```python
from build123d import *

# Parameters (mm, degrees)
BOSS_EXTRUDE1_DEPTH = 20
FILLET1_R           = 5
SKETCH2_R           = 30
BOSS_EXTRUDE2_DEPTH = 5
SKETCH3_R           = 17.5
BOSS_EXTRUDE3_DEPTH = 10
SKETCH4_R           = 21.75
BOSS_EXTRUDE4_DEPTH = 10
CHAMFER1_SIZE       = 5


with BuildPart() as part:
    # Sketch1 → Boss-Extrude1 (new body)
    with BuildSketch(Plane.XY):
        with BuildLine():
            Line((-32.88854382, 29.22291236), (-27.763932023, 39.472135955))
            ThreePointArc((-27.763932023, 39.472135955), (-24.076971234, 43.506508084), (-18.819660113, 45))
            Line((-18.819660113, 45), (18.819660113, 45))
            ThreePointArc((18.819660113, 45), (24.076971234, 43.506508084), (27.763932023, 39.472135955))
            Line((27.763932023, 39.472135955), (32.88854382, 29.22291236))
            ThreePointArc((32.88854382, 29.22291236), (34.464979789, 24.873698861), (35, 20.27864045))
            Line((35, 20.27864045), (35, -20.27864045))
            ThreePointArc((35, -20.27864045), (34.464979789, -24.873698861), (32.88854382, -29.22291236))
            Line((32.88854382, -29.22291236), (27.763932023, -39.472135955))
            ThreePointArc((27.763932023, -39.472135955), (24.076971234, -43.506508084), (18.819660113, -45))
            Line((18.819660113, -45), (-18.819660113, -45))
            ThreePointArc((-18.819660113, -45), (-24.076971234, -43.506508084), (-27.763932023, -39.472135955))
            Line((-27.763932023, -39.472135955), (-32.88854382, -29.22291236))
            ThreePointArc((-32.88854382, -29.22291236), (-34.464979789, -24.873698861), (-35, -20.27864045))
            Line((-35, -20.27864045), (-35, 20.27864045))
            ThreePointArc((-35, 20.27864045), (-34.464979789, 24.873698861), (-32.88854382, 29.22291236))
        make_face()
    extrude(amount=BOSS_EXTRUDE1_DEPTH)

    # Fillet1
    fillet1_edges = [part.edges().sort_by_distance(p)[0] for p in [
        (24.076971234, -43.506508084, 20),
        (30.326237921, -34.347524158, 20),
        (34.464979789, -24.873698861, 20),
        (35, 0, 20),
        (34.464979789, 24.873698861, 20),
        (30.326237921, 34.347524158, 20),
        (24.076971234, 43.506508084, 20),
        (0, 45, 20),
        (-24.076971234, 43.506508084, 20),
        (-30.326237921, 34.347524158, 20),
        (-24.076971234, -43.506508084, 20),
        (-34.464979789, 24.873698861, 20),
        (-35, 0, 20),
        (-34.464979789, -24.873698861, 20),
        (-30.326237921, -34.347524158, 20),
        (0, -45, 20),
    ]]
    fillet(fillet1_edges, radius=FILLET1_R)

    # Sketch2 → Boss-Extrude2 (add)
    with BuildSketch(Plane.XY.offset(20)):
        Circle(SKETCH2_R)
    extrude(amount=BOSS_EXTRUDE2_DEPTH)

    # Sketch3 → Boss-Extrude3 (add)
    with BuildSketch(Plane.XY.offset(25)):
        Circle(SKETCH3_R)
    extrude(amount=BOSS_EXTRUDE3_DEPTH)

    # Sketch4 → Boss-Extrude4 (add)
    with BuildSketch(Plane.XY.offset(35)):
        Circle(SKETCH4_R)
    extrude(amount=BOSS_EXTRUDE4_DEPTH)

    # Chamfer1
    # the kernel refuses this chamfer: 5 mm, written as the material it adds along each edge
    with BuildSketch(Plane(origin=(0, 0, 35), x_dir=(1, 0, 0), z_dir=(0, -1, 0))) as chamfer1_piece_1_section:
        Polygon((17.5 + CHAMFER1_SIZE, 0), (17.5, -CHAMFER1_SIZE), (17.5, 0), align=None)
    chamfer1_piece_1 = revolve(axis=Axis((0, 0, 35), (0, 0, 1)), mode=Mode.PRIVATE)
    chamfer1_piece_1 = chamfer1_piece_1 & Plane(origin=(0, 0, 32.136850645), x_dir=(1, 0, 0), z_dir=(0, 0, -1)) * Cylinder(21.75, 91, mode=Mode.PRIVATE)
    add(chamfer1_piece_1)


solid = part.part
```
Source: CAD feature listing. Evaluate the final solid. Frame: model axes, mm. A direction names the side the tool comes from. Round coordinates to 2 decimals unless told otherwise and drop trailing zeros. Order: outer loops, then holes, each group sorted by start corner. A loop starts at its lowest first (then second) coordinate and runs counter-clockwise, first axis right, second up. Notation, with made-up numbers: (-8, 32) -> (19, 32) arc R31 ccw to (19, 62) -> close; hole circle Ø3 at (-4, -18). An arc over 180 degrees is marked (long way). One line per item, written item: value. Start each with the question number.
Q1. Draft query along Z for faces 1 (the flat face through (13, -13, 25)), 2 (the flat face through (0, -45, 7)), 3 (the conical face through (16.89, 5.32, 30.21)), 4 (the cylindrical face through (34, 0, 18)). Return one class per face: pulls with the +Z half, pulls with the -Z half, needs draft (parallel to the pull), parting line crosses it, or undercut.
Q2. Access query for faces 5 (the flat face through (0, 0, 45)), 6 (the flat face through (2.4, -30.3, 20)). Directions: +Z, -Z, +X, -X, +Y, -Y. A direction counts if a zero-diameter tool reaches every point of the face in a straight line with its end or side. Return the directions, or none.
Q3. Section query A-A (x = 0). Return the cut outline in (y, z), plus the area to 3 significant figures.
Q4. Pin query (flat end, axial travel): pin 1 (4 mm diameter, centred on y = -12.5, z = 39.5, fed in from +X); pin 2 (12 mm diameter, centred on y = 35, z = 21.5, fed in from +X); pin 3 (5 mm diameter, centred on y = 9, z = 23.5, fed in from +X). Return the tip coordinate at first contact, or that it passes through.
Q5. Section query B-B (z = 29). Return the cut outline in (x, y), plus the area to 3 significant figures.
Q6. Material intervals for probe 1 along Z at (x, y) = (-12, 32.5); probe 2 along Z at (x, y) = (-27, 9); probe 3 along Y at (x, z) = (-14, 18.5), sorted ascending.
Findings below:
1. face 1: undercut
1. face 2: needs draft
1. face 3: undercut
1. face 4: pulls with the +Z half
2. face 5: +Z, +X, -X, +Y, -Y
2. face 6: +Z, -Y
3. outline: (-45, 0) -> (45, 0) -> (45, 15) arc R5 ccw to (40, 20) -> (30, 20) -> (30, 25) -> (17.5, 25) -> (17.5, 30) -> (21.75, 34.25) -> (21.75, 45) -> (-21.75, 45) -> (-21.75, 34.25) -> (-17.5, 30) -> (-17.5, 25) -> (-30, 25) -> (-30, 20) -> (-40, 20) arc R5 ccw to (-45, 15) -> close
3. area: 2,900 mm²
4. pin 1: x = 19.05
4. pin 2: x = 31.52
4. pin 3: x = 29.29
5. outline: circle Ø35 at (0, 0)
5. area: 962 mm²
6. probe 1: 0 to 20
6. probe 2: 0 to 25
6. probe 3: -43.57 to 43.57
